Read the model definition and answer for the solid it produces. Units are mm, in the model's axes. Give positions to 0.01 mm unless a question says otherwise; leave off trailing zeros. Order: outer loops, then holes, each group sorted by start corner. A loop starts at its lowest first (then second) coordinate and runs counter-clockwise, first axis right, second up.
Item 1: Find the intervals of material crossed by line 1 along Y through (x, z) = (0.5, -0.6); line 2 along Y through (x, z) = (0, -0.4); line 3 along X through (y, z) = (1, 0.35), in increasing order.
Item 2: A cutting plane is placed at D-D (x = -6.25). Write down the section's boundary in (y, z).
Item 3: The mould has two halves that part along X. Classify faces 1 (the face through (-0.29, -1.32, -0.02)), 2 (the face through (-15.51, -5.85, 0.02)), 3 (the face through (-6.35, -6.177, 0.021)): +X half, -X half, draft (parallel to the pull), parting line (faces both ways), or undercut.
Item 4: Given pin 1 Ø2.5 at (x, y) = (0, 0) entering from +Z, flat-ended and moving along its own axis, determine where the tip first touches the part or whether it passes through.
Item 5: A cutting plane is placed at A-A (x = 0.5). Write down the section's boundary in (y, z).
Item 6: A cutting plane is placed at C-C (z = -1.25). Write down the section's boundary in (x, y).
Item 7: A cutting plane is placed at B-B (y = 0). Write down the section's boundary in (x, z).
from build123d import *

# Parameters (mm, degrees)
SKETCH1_R  = 1.35
PAWL_DEPTH = 1.5


with BuildPart() as part:
    # Sketch1 → Pawl (new, symmetric)
    with BuildSketch(Plane.XY):
        with BuildLine():
            Line((0.824491602, 2.884478046), (0, 3))
            ThreePointArc((0, 3), (-1.377173166, 2.665219329), (-2.446979028, 1.735596047))
            ThreePointArc((-2.446979028, 1.735596047), (-8.376740645, -3.335986631), (-16, -5))
            Line((-16, -5), (-15, -6.732050808))
            ThreePointArc((-15, -6.732050808), (-6.23012531, -6.146721639), (1.740902704, -2.443206454))
            ThreePointArc((1.740902704, -2.443206454), (2.956580376, 0.508559221), (0.824491602, 2.884478046))
        make_face()
        Circle(SKETCH1_R, mode=Mode.SUBTRACT)
    extrude(amount=PAWL_DEPTH, both=True)


solid = part.part
Response values:
1. line 1: y = -3.27 to -1.25, 1.25 to 2.93
1. line 2: y = -3.57 to -1.35, 1.35 to 3
1. line 3: x = -3 to -0.91, 0.91 to 2.83
2. outline: (-6.15, -1.5) - (-2.06, -1.5) - (-2.06, 1.5) - (-6.15, 1.5) - close
3. face 1: undercut
3. face 2: -X half
3. face 3: parting line
4. pin 1: passes through
5. outline: (-3.27, -1.5) - (-1.25, -1.5) - (-1.25, 1.5) - (-3.27, 1.5) - close; (1.25, -1.5) - (2.93, -1.5) - (2.93, 1.5) - (1.25, 1.5) - close
6. outline: (-16, -5) - (-15, -6.73) arc R24 ccw to (1.74, -2.44) arc R3 ccw to (0.82, 2.88) - (0, 3) arc R3 ccw to (-2.45, 1.74) arc R16 cw to start; hole circle Ø2.7 at (0, 0)
7. outline: (-3.87, -1.5) - (-1.35, -1.5) - (-1.35, 1.5) - (-3.87, 1.5) - close; (1.35, -1.5) - (3, -1.5) - (3, 1.5) - (1.35, 1.5) - close
